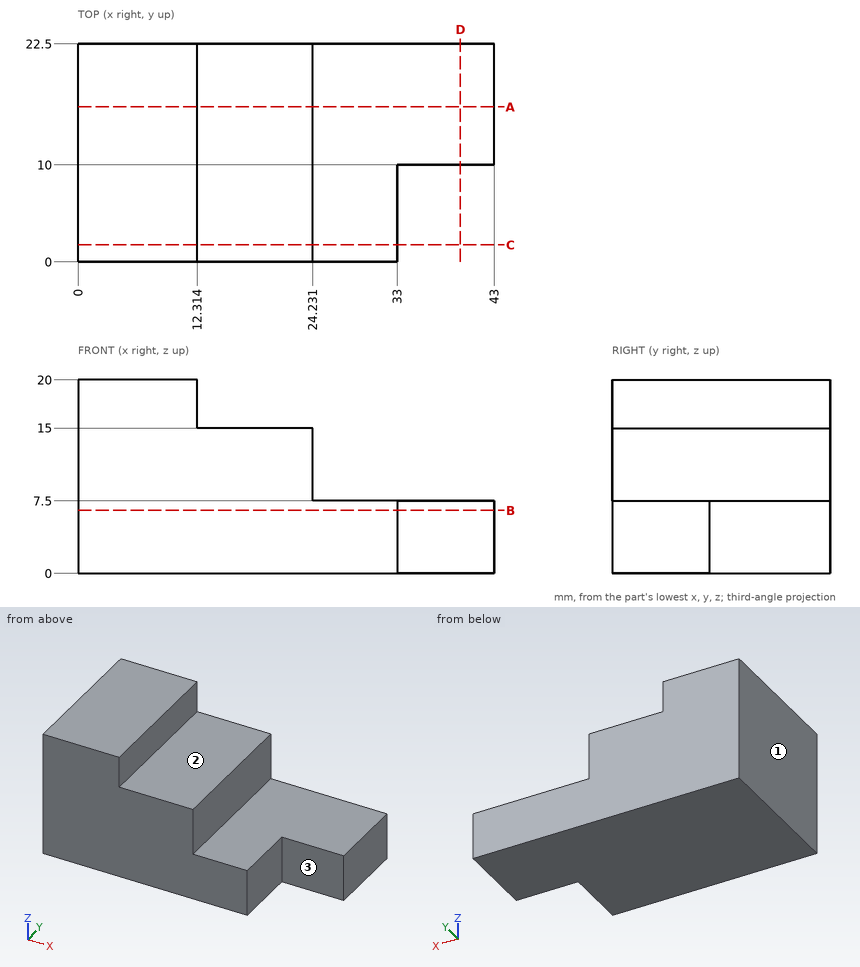
Can you work these out from the drawing? Everything is in mm from the part's minimum corner. A direction names the side the tool comes from. Give positions to 0.01 mm unless a question says otherwise; leave off trailing zeros. Loops run counter-clockwise (first coordinate to the right, second up) from the corner with the lowest first, then second, coordinate; pieces in that order, holes last. Notation, with made-up numbers: M 51.25,60 L 62.25,60 A25 cw 62.25,87 Z; hole C 89.25,-12 d2. An arc over 180 degrees is marked long. Put each result on its own line as item: value. Start each with the question number.
(1) Will these pins go through, and if not, where does the flat tip stop? pin 1 Ø2 at (y, z) = (9, 10) entering from +X; pin 2 Ø2 at (x, z) = (39.5, 4.5) entering from -Y; pin 3 Ø4 at (y, z) = (14.5, 18.5) entering from +X.
(2) I want a section at C-C on y = 1.75. Please give me the cut outline in (x, z), then the cut area to 3 significant figures.
(3) I want a section at A-A on y = 16. Please give me the cut outline in (x, z).
(4) I want a section at B-B on z = 6.5. Please give me the cut outline in (x, y).
(5) I need wall thicknesses on line 1 along Z through (x, y) = (13, 11.25); line 2 along X through (y, z) = (16.75, 7.75); line 3 along Z through (x, y) = (31, 17.5). Which ranges of each line are inside material? Lowest first, please. Write a range as [from, to].
(6) I want a section at D-D on x = 39.5. Please give me the cut outline in (y, z).
(7) For the marked faces 1, 2 and 3, which set-ups out of +Z, -Z, +X, -X, +Y, -Y let a thin tool reach every point of the face, with its end or its side?
Answer block:
1. pin 1: x = 24.23
1. pin 2: y = 10
1. pin 3: x = 12.31
2. outline: M 0,0 L 33,0 L 33,7.5 L 24.23,7.5 L 24.23,15 L 12.31,15 L 12.31,20 L 0,20 Z
2. area: 491 mm^2
3. outline: M 0,0 L 43,0 L 43,7.5 L 24.23,7.5 L 24.23,15 L 12.31,15 L 12.31,20 L 0,20 Z
4. outline: M 0,0 L 33,0 L 33,10 L 43,10 L 43,22.5 L 0,22.5 Z
5. line 1: [0, 15]
5. line 2: [0, 24.23]
5. line 3: [0, 7.5]
6. outline: M 10,0 L 22.5,0 L 22.5,7.5 L 10,7.5 Z
7. face 1: +Z, -Z, -X, +Y, -Y
7. face 2: +Z, +X, +Y, -Y
7. face 3: +Z, -Z, +X, -Y
